Here's how the part is built. I have some questions about the finished solid (model axes, mm). Face numbers are marked on the shaded views. Give positions to 0.01 mm unless a question says otherwise; leave off trailing zeros. Write each loop counter-clockwise with the first axis right and the second up, starting at its lowest first coordinate (ties: lowest second). Pieces come first, ordered by that corner, then holes. Notation, with made-up numbers: (26.25, -9) -> (43.25, -9) arc R15 cw to (43.25, 9) -> close; hole circle Ø4 at (-7, -36.75). An arc over 180 degrees is marked (long way). Put each result on its own line as item: value. Start each with the question number.
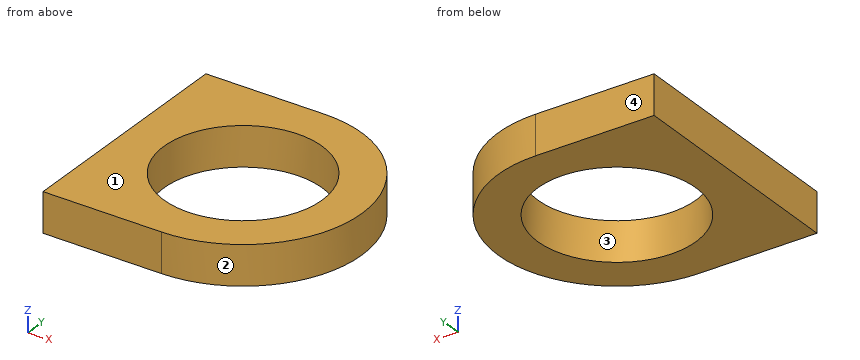
from build123d import *

# Parameters (mm, degrees)
F0_R     = 6.35
F1_DEPTH = 3.175


with BuildPart() as f1:
    # F0 (on Top) → F1 (new body)
    with BuildSketch(Plane.XY):
        with BuildLine():
            Line((0, 9.525), (0, -9.525))
            Line((0, -9.525), (9.525, -9.525))
            ThreePointArc((9.525, -9.525), (19.05, 0), (9.525, 9.525))
            Line((9.525, 9.525), (0, 9.525))
        make_face()
        with Locations((9.525, 0)):
            Circle(F0_R, mode=Mode.SUBTRACT)
    extrude(amount=F1_DEPTH)


solid = f1.part
1) Thinking about a two-plate mould opening in Y: for the marked faces 1, 2, 3 and 4, which applies, released by +Y, released by -Y, zero draft, split by the parting line, or undercut?
2) I want a section at B-B, the plane z = 0.3. Write out the boundary of the cut face in (x, y) (3 decimals), and give its area (3 significant figures).
3) I want a section at A-A, the plane y = 0. Write out the boundary of the cut face in (x, z) (3 decimals).
4) I want a section at D-D, the plane x = 17.75. Write out the boundary of the cut face in (y, z) (3 decimals).
5) I need wall thicknesses on probe 1 along X at (y, z) = (0.5, 1.1); probe 2 along Y at (x, z) = (11.25, 0.2); probe 3 along Y at (x, z) = (12, 2.05). Which ranges of each line are inside material? Lowest first, please.
6) I want a section at C-C, the plane x = 8.25. Write out the boundary of the cut face in (y, z) (3 decimals).
Established:
1. face 1: zero draft
1. face 2: split by the parting line
1. face 3: undercut
1. face 4: released by +Y
2. outline: (0, -9.525) -> (9.525, -9.525) arc R9.525 ccw to (9.525, 9.525) -> (0, 9.525) -> close; hole circle Ø12.7 at (9.525, 0)
2. area: 197 mm2
3. outline: (0, 0) -> (3.175, 0) -> (3.175, 3.175) -> (0, 3.175) -> close; (15.875, 0) -> (19.05, 0) -> (19.05, 3.175) -> (15.875, 3.175) -> close
4. outline: (-4.804, 0) -> (4.804, 0) -> (4.804, 3.175) -> (-4.804, 3.175) -> close
5. probe 1: x = 0 to 3.19, 15.86 to 19.04
5. probe 2: y = -9.37 to -6.11, 6.11 to 9.37
5. probe 3: y = -9.2 to -5.85, 5.85 to 9.2
6. outline: (-9.525, 0) -> (-6.221, 0) -> (-6.221, 3.175) -> (-9.525, 3.175) -> close; (6.221, 0) -> (9.525, 0) -> (9.525, 3.175) -> (6.221, 3.175) -> close
